```python
from build123d import *

# Parameters (mm, degrees)
BOX001_W     = 10
BOX001_H     = 10
BOX001_DEPTH = 10
BOX_W        = 10
BOX_H        = 10
BOX_DEPTH    = 10


with BuildPart() as cubo001:
    # Box001 → Box001 (new body)
    with BuildSketch(Plane(origin=(7, 7, 0), x_dir=(1, 0, 0), z_dir=(0, 0, 1))):
        with Locations((5, 5)):
            Rectangle(BOX001_W, BOX001_H)
    extrude(amount=BOX001_DEPTH)


with BuildPart() as fusion:
    # Box → Box (new body)
    with BuildSketch(Plane.XY):
        with Locations((5, 5)):
            Rectangle(BOX_W, BOX_H)
    extrude(amount=BOX_DEPTH)

    # Fusion: union Cubo001
    add(cubo001.part)


solid = fusion.part
```
Input: part model. Units: mm. Frame: model coordinates. A direction names the side the tool comes from. Give positions to 0.01 mm unless a question says otherwise; leave off trailing zeros. Write each loop counter-clockwise with the first axis right and the second up, starting at its lowest first coordinate (ties: lowest second). Pieces come first, ordered by that corner, then holes. Notation, with made-up numbers: (29.5, -35) - (44.5, -35) arc R24 cw to (44.5, -1) - close; hole circle Ø6 at (31.5, -33.75). An arc over 180 degrees is marked (long way). Write item = value, one per line. Start each with the question number.
1) Reachability of faces 1 (the face through (3, 10, 5)), 2 (the face through (12, 17, 5)), 3 (the face through (10, 3, 5)) from +Z, -Z, +X, -X, +Y, -Y: full face, straight path, thin tool, end or side. Return the list, or none.
2) Material intervals for L1, parallel to Y at x = 14.5, z = 9; L2, parallel to X at y = 6.5, z = 4.5, sorted ascending. Write a range as [from, to].
3) Cut plane B-B (x = 12.75). Return loops of the section in (y, z), and give its area (3 significant figures).
4) Cut plane A-A (z = 9). Return loops of the section in (x, y), and give its area (3 significant figures).
5) Pin query (flat end, axial travel): pin 1 (3.5 mm diameter, centred on y = 3, z = 5, fed in from +X); pin 2 (6 mm diameter, centred on y = 15, z = 4, fed in from -X); pin 3 (5.5 mm diameter, centred on x = 15, z = 3.5, fed in from -Y). Return the tip coordinate at first contact, or that it passes through.
Answers follow:
q1.face_1 = +Z, -Z, -X, +Y
q1.face_2 = +Z, -Z, +X, -X, +Y
q1.face_3 = +Z, -Z, +X, -Y
q2.L1 = [7, 17]
q2.L2 = [0, 10]
q3.outline = (7, 0) - (17, 0) - (17, 10) - (7, 10) - close
q3.area = 100 mm^2
q4.outline = (0, 0) - (10, 0) - (10, 7) - (17, 7) - (17, 17) - (7, 17) - (7, 10) - (0, 10) - close
q4.area = 191 mm^2
q5.pin_1 = 10
q5.pin_2 = 7
q5.pin_3 = 7
